```python
from build123d import *

# Parameters (mm, degrees)
SKETCH1_W                 = 50.8
SKETCH1_H                 = 127
BOSS_EXTRUDE1_DEPTH       = 3.175
SKETCH2_W                 = 3.175
SKETCH2_H                 = 25.4
CUT_EXTRUDE1_DEPTH        = 3.175
LPATTERN1_COUNT           = 2
LPATTERN1_PITCH           = 50.8
LPATTERN2_COUNT           = 2
LPATTERN2_PITCH           = 50.8
SKETCH3_W                 = 3.175
SKETCH3_H                 = 25.4
CUT_EXTRUDE2_DEPTH        = 3.175
LPATTERN3_COUNT           = 2
LPATTERN3_PITCH           = 50.8
LPATTERN4_COPY_1_SKETCH_W = 3.175
LPATTERN4_COPY_1_SKETCH_H = 25.4
LPATTERN4_COPY_1_DEPTH    = 3.175
LPATTERN4_COPY_2_SKETCH_W = 3.175
LPATTERN4_COPY_2_SKETCH_H = 25.4
LPATTERN4_COPY_2_DEPTH    = 3.175
SKETCH6_W                 = 10.205647586
SKETCH6_H                 = 3.175
CUT_EXTRUDE3_DEPTH        = 3.175
LPATTERN5_COUNT           = 2
LPATTERN5_PITCH           = 20.32


with BuildPart() as part:
    # Sketch1 → Boss-Extrude1 (new body)
    with BuildSketch(Plane(origin=(0, 0, 0), x_dir=(1, 0, 0), z_dir=(0, 1, 0))):
        Rectangle(SKETCH1_W, SKETCH1_H)
    extrude(amount=BOSS_EXTRUDE1_DEPTH)

    # Sketch2 → Cut-Extrude1 (cut)
    with BuildSketch(Plane(origin=(0, 3.175, 0), x_dir=(1, 0, 0), z_dir=(0, 1, 0))):
        with Locations((-23.8125, 0)):
            Rectangle(SKETCH2_W, SKETCH2_H)
    cut_extrude1 = extrude(amount=-CUT_EXTRUDE1_DEPTH, mode=Mode.SUBTRACT)

    # LPattern1: Cut-Extrude1 ×2
    with Locations(*[(0, 0, -i * LPATTERN1_PITCH) for i in range(1, LPATTERN1_COUNT)]):
        add(cut_extrude1, mode=Mode.SUBTRACT)

    # LPattern2: Cut-Extrude1 ×2
    with Locations(*[(0, 0, i * LPATTERN2_PITCH) for i in range(1, LPATTERN2_COUNT)]):
        add(cut_extrude1, mode=Mode.SUBTRACT)

    # Sketch3 → Cut-Extrude2 (cut)
    with BuildSketch(Plane(origin=(0, 3.175, 0), x_dir=(1, 0, 0), z_dir=(0, 1, 0))):
        with Locations((23.8125, 50.8)):
            Rectangle(SKETCH3_W, SKETCH3_H)
    cut_extrude2 = extrude(amount=-CUT_EXTRUDE2_DEPTH, mode=Mode.SUBTRACT)

    # LPattern3: Cut-Extrude2 ×2
    with Locations(*[(0, 0, i * LPATTERN3_PITCH) for i in range(1, LPATTERN3_COUNT)]):
        add(cut_extrude2, mode=Mode.SUBTRACT)

    # LPattern4 copy 1 sketch → LPattern4 copy 1 (cut)
    with BuildSketch(Plane(origin=(0, 3.175, 101.6), x_dir=(1, 0, 0), z_dir=(0, 1, 0))):
        with Locations((23.8125, 50.8)):
            Rectangle(LPATTERN4_COPY_1_SKETCH_W, LPATTERN4_COPY_1_SKETCH_H)
    extrude(amount=-LPATTERN4_COPY_1_DEPTH, mode=Mode.SUBTRACT)

    # LPattern4 copy 2 sketch → LPattern4 copy 2 (cut)
    with BuildSketch(Plane(origin=(0, 3.175, 50.8), x_dir=(1, 0, 0), z_dir=(0, 1, 0))):
        with Locations((23.8125, 50.8)):
            Rectangle(LPATTERN4_COPY_2_SKETCH_W, LPATTERN4_COPY_2_SKETCH_H)
    extrude(amount=-LPATTERN4_COPY_2_DEPTH, mode=Mode.SUBTRACT)

    # Sketch6 → Cut-Extrude3 (cut)
    with BuildSketch(Plane(origin=(0, 3.175, 0), x_dir=(1, 0, 0), z_dir=(0, 1, 0))):
        with Locations((10.182823793, 61.9125)):
            Rectangle(SKETCH6_W, SKETCH6_H)
        with Locations((10.182823793, -61.9125)):
            Rectangle(SKETCH6_W, SKETCH6_H)
    cut_extrude3 = extrude(amount=-CUT_EXTRUDE3_DEPTH, mode=Mode.SUBTRACT)

    # LPattern5: Cut-Extrude3 ×2
    with Locations(*[(-i * LPATTERN5_PITCH, 0, 0) for i in range(1, LPATTERN5_COUNT)]):
        add(cut_extrude3, mode=Mode.SUBTRACT)


solid = part.part
```
CAD build for the part. Positions are in the model's coordinates, mm. A direction names the side the tool comes from. Coordinates: 2 decimals unless noted, no trailing zeros. Loops run counter-clockwise (first coordinate to the right, second up) from the corner with the lowest first, then second, coordinate; pieces in that order, holes last. Notation, with made-up numbers: (88.25, 47) - (93.25, 47) arc R23 ccw to (93.25, 82) - close; hole circle Ø2 at (1.25, 10). An arc over 180 degrees is marked (long way). Use CSV: the item, a comma, the result in double quotes. Start each with the question number.
Q1. Cut at A-A, the plane x = 12.5. List the corners of the cut face in (y, z) (3 decimals).
Q2. Probe probe 1 along Z at (x, y) = (23.5, 2.35); probe 2 along Z at (x, y) = (11, 1.35) (3 decimals); probe 3 along X at (y, z) = (1.9, -11) (3 decimals). List the from-to ranges inside material, lowest first. Write a range as from..to.
Q3. 3-axis set-ups, long thin cutter, end or side, ignore diameter. For faces 1 (the flat face through (22.225, 2, 51)), 2 (the flat face through (24, 2, -12.7)), 3 (the flat face through (-24, 2, -38.1)), 4 (the flat face through (15.286, 2, 62)), 5 (the flat face through (10, 2, -60.325)): which of +Z, -Z, +X, -X, +Y, -Y reach the whole face in a straight line?
Q4. Drop flat-ended pins along their axis: P1, Ø1, axis at x = 24, y = 1.5, coming from the -Z side; P2, Ø1.6, axis at y = 1, z = 0, coming from the -X side (3 decimals); P3, Ø1.6, axis at y = 1, z = 61.5, coming from the +X side (3 decimals). Give the stop position or say it passes through.
Q5. Cut at B-B, the plane z = 53. List the corners of the cut face in (x, y) (3 decimals), then the cut area to 3 significant figures.
Q6. Two-plate mould, pull along X, no slides. Class faces 6 (the flat face through (-22.225, 2, 0)), 7 (the flat face through (-24, 2, -12.7)), 8 (the flat face through (25.4, 2, -25)), 9 (the flat face through (-15.24, 2, -62)): +X half, -X half, draft (parallel to the pull), parting line (faces both ways), or undercut.
Here are the results:
1,outline,"(0, -60.325) - (3.175, -60.325) - (3.175, 60.325) - (0, 60.325) - close"
2,probe 1,"-38.1..-12.7, 12.7..38.1"
2,probe 2,"-60.325..60.325"
2,probe 3,"-22.225..22.225"
3,face 1,"+Z, +X, +Y, -Y"
3,face 2,"+X, +Y, -Y"
3,face 3,"-Z, -X, +Y, -Y"
3,face 4,"+Z, +Y, -Y"
3,face 5,"-Z, +Y, -Y"
4,P1,"z = -38.1"
4,P2,"x = -22.225"
4,P3,"x = 22.225"
5,outline,"(-22.225, 0) - (22.225, 0) - (22.225, 3.175) - (-22.225, 3.175) - close"
5,area,"141 mm2"
6,face 6,"-X half"
6,face 7,"draft"
6,face 8,"+X half"
6,face 9,"undercut"
